```python
from build123d import *

# Parameters (mm, degrees)
SKETCH202_R     = 1.4
PAD127038_DEPTH = 10
PAD127037_DEPTH = 1
PAD127010_DEPTH = 26


with BuildPart() as setscrewcutout:
    # Sketch202 → Pad127038 (new body, symmetric)
    with BuildSketch(Plane(origin=(75, 0, 0), x_dir=(1, 0, 0), z_dir=(0, -1, 0))):
        with Locations((-22.5, 0)):
            Circle(SKETCH202_R)
    extrude(amount=PAD127038_DEPTH, both=True)


with BuildPart() as endcap:
    # Sketch201 → Pad127037 (new body)
    with BuildSketch(Plane.YZ.offset(75)):
        Polygon((8, 4.618802), (0, 9.237604), (-8, 4.618802), (-8, -4.618802), (0, -9.237604), (8, -4.618802), align=None)
        Polygon((0, 5.5), (-4.76314, 2.75), (-4.76314, -2.75), (0, -5.5), (4.76314, -2.75), (4.76314, 2.75), align=None, mode=Mode.SUBTRACT)
    extrude(amount=PAD127037_DEPTH)


with BuildPart() as wheelaxle:
    # Sketch172 → Pad127010 (new body)
    with BuildSketch(Plane.YZ.offset(75)):
        Polygon((6, 3.464102), (0, 6.928203), (-6, 3.464102), (-6, -3.464102), (0, -6.928203), (6, -3.464102), align=None)
        Polygon((0, 5.5), (-4.76314, 2.75), (-4.76314, -2.75), (0, -5.5), (4.76314, -2.75), (4.76314, 2.75), align=None, mode=Mode.SUBTRACT)
    extrude(amount=-PAD127010_DEPTH)

    # Fusion004020027: union EndCap
    add(endcap.part)

    # Cut007019023: cut SetScrewCutout
    add(setscrewcutout.part, mode=Mode.SUBTRACT)


solid = wheelaxle.part
```
Work out the finished part from the listing and answer in its coordinate system (mm). A direction names the side the tool comes from. Give positions to 0.01 mm unless a question says otherwise; leave off trailing zeros. Order: outer loops, then holes, each group sorted by start corner. A loop starts at its lowest first (then second) coordinate and runs counter-clockwise, first axis right, second up. Notation, with made-up numbers: M 29.5,52 L 38.5,52 A17 ccw 38.5,71 Z; hole C 20.5,49.5 d5. An arc over 180 degrees is marked long. Return JSON: item names as keys, results as strings.
1) Section C-C, the plane y = -3.75 is taken. Write down the section's boundary in (x, z).
Resolved:
{"outline": "M 49,-4.76 L 75,-4.76 L 75,-7.07 L 76,-7.07 L 76,-3.33 L 49,-3.33 Z; M 49,3.33 L 76,3.33 L 76,7.07 L 75,7.07 L 75,4.76 L 49,4.76 Z"}
2) Straight lines are drawn through the part: line 1 along Y through (x, z) = (70.75, -2); line 2 along X through (y, z) = (-5.25, -5.25); line 3 along Y through (x, z) = (51, -3.5). For each, find the intervals that lie inside material, in ascending order. Write a range as [from, to].
Resolved:
{"line 1": "[-6, -4.76], [4.76, 6]", "line 2": "[75, 76]", "line 3": "[-5.94, -3.46], [3.46, 5.94]"}
3) Section B-B, the plane z = 0 is taken. Write down the section's boundary in (x, y).
Resolved:
{"outline": "M 49,-6 L 51.1,-6 L 51.1,-4.76 L 49,-4.76 Z; M 49,4.76 L 51.1,4.76 L 51.1,6 L 49,6 Z; M 53.9,-6 L 75,-6 L 75,-8 L 76,-8 L 76,-4.76 L 53.9,-4.76 Z; M 53.9,4.76 L 76,4.76 L 76,8 L 75,8 L 75,6 L 53.9,6 Z"}
4) A tool of negligible diameter and unlimited length cuts with its end or side. For faces 5 (the flat face through (62.18, -2.96, 5.22)), 6 (the flat face through (62.31, -2.41, -4.11)), 7 (the flat face through (62, -6, 0)), from which of +Z, -Z, +X, -X, +Y, -Y can it reach the whole face along a straight path? Write none if from no direction.
Resolved:
{"face 5": "+Z, -X, -Y", "face 6": "+X, -X", "face 7": "+Z, -Z, -X, -Y"}
5) Each of these flat-tipped pins is pushed along its axis until it touches: pin 1 (2 mm diameter, centred on x = 62.5, z = 7, fed in from -Y); pin 2 (5 mm diameter, centred on x = 66.5, y = 1, fed in from -Z); pin 3 (1 mm diameter, centred on x = 55.5, z = 1.5, fed in from -Y); pin 4 (1.7 mm diameter, centred on x = 52.5, z = 0, fed in from +Y). Where does it stop, or does it pass through?
Resolved:
{"pin 1": "y = -1.61", "pin 2": "z = -6.93", "pin 3": "y = -6", "pin 4": "through"}
6) Section D-D, the plane z = -5 is taken. Write down the section's boundary in (x, y).
Resolved:
{"outline": "M 49,-3.34 L 75,-3.34 L 75,-7.34 L 76,-7.34 L 76,-0.87 L 49,-0.87 Z; M 49,0.87 L 76,0.87 L 76,7.34 L 75,7.34 L 75,3.34 L 49,3.34 Z"}
7) For a pull along Y with two mould halves and no side action, classify faces 1 (the flat face through (75.493, 4.056, 6.896)), 2 (the cylindrical face through (53.835, 5.373, 0.421)), 3 (the flat face through (62, 4.763, 0)), 4 (the flat face through (62, -4.763, 0)) as +Y half, -Y half, draft (parallel to the pull), parting line (faces both ways), or undercut.
Resolved:
{"face 1": "+Y half", "face 2": "draft", "face 3": "undercut", "face 4": "undercut"}
8) Section A-A, the plane x = 52.5 is taken. Write down the section's boundary in (y, z).
Resolved:
{"outline": "M -6,-3.46 L 0,-6.93 L 6,-3.46 L 6,-1.4 L 4.76,-1.4 L 4.76,-2.75 L 0,-5.5 L -4.76,-2.75 L -4.76,-1.4 L -6,-1.4 Z; M -6,1.4 L -4.76,1.4 L -4.76,2.75 L 0,5.5 L 4.76,2.75 L 4.76,1.4 L 6,1.4 L 6,3.46 L 0,6.93 L -6,3.46 Z"}
